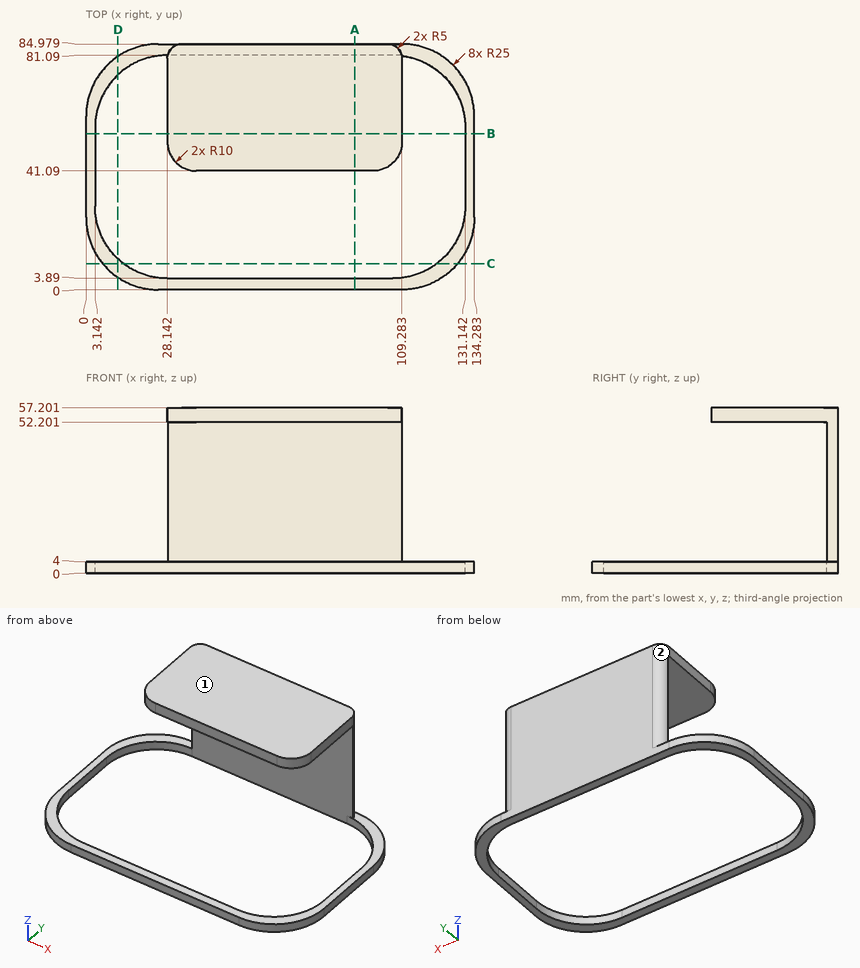
Design review of the part shown in the three views and the two pictorial views. Dimensions are in mm from the part's minimum x, y and z. A direction names the side the tool comes from. Coordinates: 2 decimals unless noted, no trailing zeros. Order: outer loops, then holes, each group sorted by start corner. A loop starts at its lowest first (then second) coordinate and runs counter-clockwise, first axis right, second up.
1) For the marked faces 1 and 2, list the 3-axis set-ups (+Z, -Z, +X, -X, +Y, -Y) from which the entire face can be reached by the end or side of a thin tool; tool diameter is ignored.
2) Clearance check with flat-ended pins moving along their axes: pin 1 (4 mm diameter, centred on y = 59.5, z = 55, fed in from +X); pin 2 (1.5 mm diameter, centred on x = 66, z = 55, fed in from -Y); pin 3 (3 mm diameter, centred on x = 59.5, y = 38.5, fed in from -Z); pin 4 (20 mm diameter, centred on x = 84.5, y = 64, fed in from -Z). State where each tip first meets the part, or that it passes through.
3) Take a section at D-D, the plane x = 11. Give the boundary of the cut face in (y, z).
4) Wall thickness on line 1 along Z through (x, y) = (84.5, 51.5); line 2 along Y through (x, z) = (61.5, 35); line 3 along Z through (x, y) = (7.5, 11.5): over which ranges is each line inside the solid? List them lowest first.
5) Take a section at B-B, the plane y = 54. Give the boundary of the cut face in (x, z).
6) Take a section at C-C, the plane y = 9. Give the boundary of the cut face in (x, z) (1 decimal).
7) Take a section at A-A, the plane x = 93. Give the boundary of the cut face in (y, z).
Returned:
1. face 1: +Z, +X, -X, +Y, -Y
1. face 2: +Z, -X, +Y
2. pin 1: stops at x = 109.28
2. pin 2: stops at y = 41.09
2. pin 3: passes through
2. pin 4: stops at z = 52.2
3. outline: (4.29, 0) - (10.69, 0) - (10.69, 4) - (4.29, 4) - close; (74.29, 0) - (80.69, 0) - (80.69, 4) - (74.29, 4) - close
4. line 1: z = 52.2 to 57.2
4. line 2: y = 81.09 to 84.98
4. line 3: z = 0 to 4
5. outline: (0, 0) - (3.14, 0) - (3.14, 4) - (0, 4) - close; (28.14, 52.2) - (109.28, 52.2) - (109.28, 57.2) - (28.14, 57.2) - close; (131.14, 0) - (134.28, 0) - (134.28, 4) - (131.14, 4) - close
6. outline: (5.8, 0) - (13, 0) - (13, 4) - (5.8, 4) - close; (121.3, 0) - (128.5, 0) - (128.5, 4) - (121.3, 4) - close
7. outline: (0, 0) - (3.89, 0) - (3.89, 4) - (0, 4) - close; (41.09, 52.2) - (81.09, 52.2) - (81.09, 0) - (84.98, 0) - (84.98, 57.2) - (41.09, 57.2) - close
